Input: part model. Units: mm. Frame: model coordinates. Face numbers are marked on the shaded views. A direction names the side the tool comes from. Coordinates: 2 decimals unless noted, no trailing zeros. Order: outer loops, then holes, each group sorted by start corner. A loop starts at its lowest first (then second) coordinate and runs counter-clockwise, first axis right, second up. Notation, with made-up numbers: (56, -13) - (72, -13) arc R28 cw to (72, 22) - close; hole circle Ø7 at (89.5, 81.25). An arc over 180 degrees is marked (long way). Answer as CSV lines item,"result". Start each with the question number.
Item 1: Section B-B (y = 18.5). Output: boundary loops of the cut face in (x, z) (3 decimals), and give its area (4 significant figures).
Item 2: Section A-A (z = 35). Output: boundary loops of the cut face in (x, y), and give its area (3 significant figures).
Item 3: First-contact query: pin 1 (1.8 mm diameter, centred on x = 7.5, y = 41, fed in from -Z); pin 2 (18 mm diameter, centred on x = 55, z = -3.5, fed in from -Y). Flat tips, straight axial feed; report the tip coordinate or a pass-through.
Item 4: Access query for the marked faces 1, 2 and 3. Directions: +Z, -Z, +X, -X, +Y, -Y. A direction counts if a zero-diameter tool reaches every point of the face in a straight line with its end or side. Return the directions, or none.
Item 5: Section C-C (z = -2). Output: boundary loops of the cut face in (x, y), and give its area (3 significant figures).
Item 6: Section D-D (x = 41). State how many separate pieces and enclosed holes the cut face has, and give its area (3 significant figures).
Item 7: Draft query along Z for the marked faces 4, 5 and 6. Return one class per face: +Z half, -Z half, draft (parallel to the pull), parting line (faces both ways), or undercut.
Item 8: Material intervals for line 1 along Y through (x, z) = (118.5, 96); line 2 along Y through (x, z) = (79.5, -20); line 3 along Z through (x, y) = (53, 55) (3 decimals), sorted ascending.
from build123d import *

# Parameters (mm, degrees)
BOSS_EXTRUDE1_DEPTH     = 126
SKETCH2_R               = 1.5
CUT_EXTRUDE1_DEPTH      = 46.25
SKETCH3_R               = 1.5
CUT_EXTRUDE3_DEPTH      = 53.75
CUT_EXTRUDE6_DEPTH      = 46.25
SKETCH5_W               = 120
SKETCH5_H               = 5
SKETCH5_H_2             = 0.575
SKETCH5_W_2             = 35.5
CUT_EXTRUDE7_DEPTH      = 188.549070389
CUT_EXTRUDE8_DEPTH      = 201.864965658
CUT_EXTRUDE8_DEPTH_BACK = 201.864965658
CUT_EXTRUDE9_DEPTH      = 203.827454511
CUT_EXTRUDE9_DEPTH_BACK = 203.827454511
SKETCH7_R               = 1.5
SKETCH8_W               = 1
SKETCH8_H               = 3.175
BOSS_EXTRUDE2_DEPTH     = 126


with BuildPart() as part:
    # Sketch1 → Boss-Extrude1 (new body)
    with BuildSketch(Plane(origin=(0, 0, 0), x_dir=(0, 0, -1), z_dir=(1, 0, 0))):
        Polygon((-95, -3.570472346), (-95, 46.429527654), (-59.5, 46.429527654), (-59.5, 50.179527654), (-95, 50.179527654), (-95, 92.679527654), (-43.5, 92.679527654), (-35, 92.679527654), (-35, 96.429527654), (-43.5, 96.429527654), (-90, 96.429527654), (-100, 96.429527654), (-100, 86.429527654), (-100, -8.570472346), (-90, -8.570472346), (-35, -8.570472346), (-35, -3.570472346), align=None)
    boss_extrude1 = extrude(amount=BOSS_EXTRUDE1_DEPTH)

    # Sketch2 → Cut-Extrude1 (cut)
    with BuildSketch(Plane(origin=(0, 96.429527654, 0), x_dir=(1, 0, 0), z_dir=(0, 1, 0))):
        with Locations(Location((3, -47.6, 0), (0, 0, 270))):
            Circle(SKETCH2_R)
        with Locations(Location((123, -47.6, 0), (0, 0, 270))):
            Circle(SKETCH2_R)
    cut_extrude1 = extrude(amount=-CUT_EXTRUDE1_DEPTH, mode=Mode.SUBTRACT)

    # Sketch3 → Cut-Extrude3 (cut)
    with BuildSketch(Plane(origin=(0, 50.179527654, 0), x_dir=(1, 0, 0), z_dir=(0, 1, 0))):
        with Locations(Location((3, -66.6, 0), (0, 0, 270))):
            Circle(SKETCH3_R)
        with Locations(Location((123, -66.6, 0), (0, 0, 270))):
            Circle(SKETCH3_R)
        with BuildLine():
            Line((6, -65), (6, -35))
            Line((6, -35), (120, -35))
            Line((120, -35), (120, -65))
            ThreePointArc((120, -65), (117.071067812, -72.071067812), (110, -75))
            Line((110, -75), (16, -75))
            ThreePointArc((16, -75), (8.928932188, -72.071067812), (6, -65))
        make_face()
    cut_extrude3 = extrude(amount=-CUT_EXTRUDE3_DEPTH, mode=Mode.SUBTRACT)

    # Mirror2: Boss-Extrude1, Cut-Extrude1, Cut-Extrude3 across plane
    add(boss_extrude1.mirror(Plane(origin=(0, 0, 35), x_dir=(1, 0, 0), z_dir=(0, 0, -1))))
    add(cut_extrude1.mirror(Plane(origin=(0, 0, 35), x_dir=(1, 0, 0), z_dir=(0, 0, -1))), mode=Mode.SUBTRACT)
    add(cut_extrude3.mirror(Plane(origin=(0, 0, 35), x_dir=(1, 0, 0), z_dir=(0, 0, -1))), mode=Mode.SUBTRACT)

    # Sketch4 → Cut-Extrude6 (cut)
    with BuildSketch(Plane(origin=(0, 96.429527654, 0), x_dir=(1, 0, 0), z_dir=(0, 1, 0))):
        with BuildLine():
            Line((9, -35), (9, -70))
            ThreePointArc((9, -70), (11.928932188, -77.071067812), (19, -80))
            Line((19, -80), (106.999682888, -80))
            ThreePointArc((106.999682888, -80), (114.0707507, -77.071067812), (116.999682888, -70))
            Line((116.999682888, -70), (116.999682888, -35))
            Line((116.999682888, -35), (9, -35))
        make_face()
    cut_extrude6 = extrude(amount=-CUT_EXTRUDE6_DEPTH, mode=Mode.SUBTRACT)

    # Mirror5: Cut-Extrude6 across plane
    add(cut_extrude6.mirror(Plane(origin=(0, 0, 35), x_dir=(1, 0, 0), z_dir=(0, 0, -1))), mode=Mode.SUBTRACT)

    # Sketch5 → Cut-Extrude7 (cut, through all)
    with BuildSketch(Plane(origin=(126, 0, 0), x_dir=(0, 0, -1), z_dir=(1, 0, 0))):
        with Locations((-35, -6.070472346)):
            Rectangle(SKETCH5_W, SKETCH5_H)
        Polygon((-100, 96.429527654), (-98.175, 96.429527654), (-97.175, 96.429527654), (-97.175, 93.254527654), (-98.175, 93.254527654), (-98.175, -8.570472346), (-100, -8.570472346), align=None)
        with Locations((-35, 92.967027654)):
            Rectangle(SKETCH5_W, SKETCH5_H_2)
        with Locations((-77.25, 46.717027654)):
            Rectangle(SKETCH5_W_2, SKETCH5_H_2)
        with Locations((7.25, 46.717027654)):
            Rectangle(SKETCH5_W_2, SKETCH5_H_2)
        Polygon((28.175, 93.254527654), (28.175, -8.570472346), (30, -8.570472346), (30, 96.429527654), (28.175, 96.429527654), (27.175, 96.429527654), (27.175, 93.254527654), align=None)
    extrude(amount=-CUT_EXTRUDE7_DEPTH, mode=Mode.SUBTRACT)

    # Sketch6 → Cut-Extrude8 (cut, two sides: drawn at the far end of the back side and taken through both)
    with BuildSketch(Plane(origin=(0, 0, 95), x_dir=(-1, 0, 0), z_dir=(0, 0, -1)).offset(-CUT_EXTRUDE8_DEPTH_BACK)):
        with BuildLine():
            Line((-100.999841444, 85.754527654), (-25, 85.754527654))
            ThreePointArc((-25, 85.754527654), (-17.928932188, 82.825595466), (-15, 75.754527654))
            Line((-15, 75.754527654), (-15, 67.679527654))
            ThreePointArc((-15, 67.679527654), (-17.928932188, 60.608459842), (-25, 57.679527654))
            Line((-25, 57.679527654), (-100.999841444, 57.679527654))
            ThreePointArc((-100.999841444, 57.679527654), (-108.070909256, 60.608459842), (-110.999841444, 67.679527654))
            Line((-110.999841444, 67.679527654), (-110.999841444, 75.754527654))
            ThreePointArc((-110.999841444, 75.754527654), (-108.070909256, 82.825595466), (-100.999841444, 85.754527654))
        make_face()
        with BuildLine():
            Line((-101, 39.504527654), (-25, 39.504527654))
            ThreePointArc((-25, 39.504527654), (-17.928932188, 36.575595466), (-15, 29.504527654))
            Line((-15, 29.504527654), (-15, 8.929527654))
            ThreePointArc((-15, 8.929527654), (-17.928932188, 1.858459842), (-25, -1.070472346))
            Line((-25, -1.070472346), (-101, -1.070472346))
            ThreePointArc((-101, -1.070472346), (-108.071067812, 1.858459842), (-111, 8.929527654))
            Line((-111, 8.929527654), (-111, 29.504527654))
            ThreePointArc((-111, 29.504527654), (-108.071067812, 36.575595466), (-101, 39.504527654))
        make_face()
    extrude(amount=CUT_EXTRUDE8_DEPTH + CUT_EXTRUDE8_DEPTH_BACK, mode=Mode.SUBTRACT)

    # Sketch7 → Cut-Extrude9 (cut, two sides: drawn at the far end of the back side and taken through both)
    with BuildSketch(Plane.XY.offset(98.175).offset(-CUT_EXTRUDE9_DEPTH_BACK)):
        with Locations((118.5, 87.254527654)):
            Circle(SKETCH7_R)
        with Locations((118.5, 56.179527654)):
            Circle(SKETCH7_R)
        with Locations((118.5, 41.004527654)):
            Circle(SKETCH7_R)
        with Locations((118.5, -2.570472346)):
            Circle(SKETCH7_R)
        with Locations(Location((7.5, -2.570472346, 0), (0, 0, 90))):
            Circle(SKETCH7_R)
        with Locations(Location((7.5, 41.004527654, 0), (0, 0, 90))):
            Circle(SKETCH7_R)
        with Locations(Location((7.5, 56.179527654, 0), (0, 0, 180))):
            Circle(SKETCH7_R)
        with Locations(Location((7.5, 87.254527654, 0), (0, 0, 180))):
            Circle(SKETCH7_R)
    extrude(amount=CUT_EXTRUDE9_DEPTH + CUT_EXTRUDE9_DEPTH_BACK, mode=Mode.SUBTRACT)

    # Sketch8 → Boss-Extrude2 (add)
    with BuildSketch(Plane(origin=(126, 0, 0), x_dir=(0, 0, -1), z_dir=(1, 0, 0))):
        with Locations((-97.675, 94.842027654)):
            Rectangle(SKETCH8_W, SKETCH8_H)
        with Locations((27.675, 94.842027654)):
            Rectangle(SKETCH8_W, SKETCH8_H)
    extrude(amount=-BOSS_EXTRUDE2_DEPTH)


solid = part.part
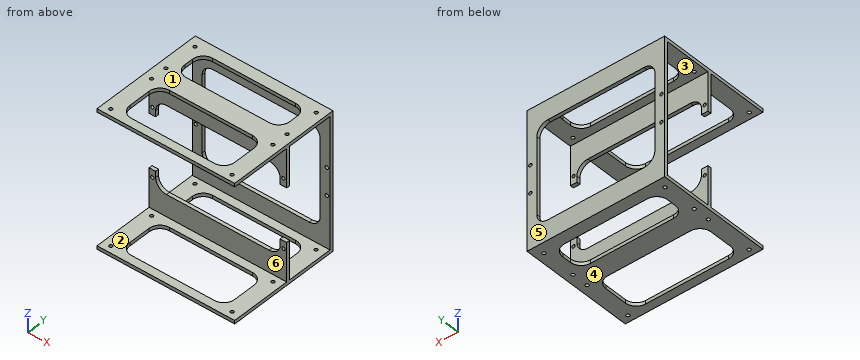
Determined:
1,outline,"(0, -28.175) - (15, -28.175) - (15, -25) - (0, -25) - close; (0, 95) - (15, 95) - (15, 98.175) - (0, 98.175) - close; (111, -28.175) - (126, -28.175) - (126, -25) - (111, -25) - close; (111, 95) - (126, 95) - (126, 98.175) - (111, 98.175) - close"
1,area,"190.5 mm^2"
2,outline,"(0, 93.25) - (9, 93.25) - (9, 96.43) - (0, 96.43) - close; (117, 93.25) - (126, 93.25) - (126, 96.43) - (117, 96.43) - close"
2,area,"57.2 mm^2"
3,pin 1,"passes through"
3,pin 2,"stops at y = 47"
4,face 1,"+Z, +X, -X, +Y, -Y"
4,face 2,"+X, -X, -Y"
4,face 3,"+X, -X"
5,outline,"(0, 47) - (8.86, 47) - (8.86, 50.18) - (0, 50.18) - close; (0, 93.25) - (9.2, 93.25) - (9.2, 96.43) - (0, 96.43) - close; (116.8, 93.25) - (126, 93.25) - (126, 96.43) - (116.8, 96.43) - close; (117.14, 47) - (126, 47) - (126, 50.18) - (117.14, 50.18) - close"
5,area,"115 mm^2"
6,separate pieces,"6"
6,enclosed holes,"0"
6,area,"453 mm^2"
7,face 4,"-Z half"
7,face 5,"draft"
7,face 6,"undercut"
8,line 1,"y = -8.57 to -4.07, -1.07 to 39.5, 42.5 to 54.68, 57.68 to 85.75, 88.75 to 96.43"
8,line 2,"y = 47 to 50.18, 93.25 to 96.43"
8,line 3,"z = -28.175 to -25, 95 to 98.175"
